```python
from build123d import *

# Parameters (mm, degrees)
F1_DEPTH  = 15.4
F3_DEPTH  = 5.4
F5_DEPTH  = 2
F6_R      = 6.7
F7_DEPTH  = 2
F9_DEPTH  = 8.7
F10_R     = 1.25
F11_DEPTH = 1
F12_R     = 2.85
F13_DEPTH = 3
F14_R     = 2.7
F15_DEPTH = 3
F16_R     = 1
F17_DEPTH = 5
F18_R     = 1.7
F18_R_2   = 1
F19_DEPTH = 3


with BuildPart() as f1:
    # F0 (on Top) → F1 (new body)
    with BuildSketch(Plane.XY):
        with BuildLine():
            Line((-22.9, -27.9), (22.9, -27.9))
            ThreePointArc((22.9, -27.9), (26.4355339059, -26.4355339059), (27.9, -22.9))
            Line((27.9, -22.9), (27.9, 22.9))
            ThreePointArc((27.9, 22.9), (26.4355339059, 26.4355339059), (22.9, 27.9))
            Line((22.9, 27.9), (-22.9, 27.9))
            ThreePointArc((-22.9, 27.9), (-26.4355339059, 26.4355339059), (-27.9, 22.9))
            Line((-27.9, 22.9), (-27.9, -22.9))
            ThreePointArc((-27.9, -22.9), (-26.4355339059, -26.4355339059), (-22.9, -27.9))
        make_face()
    extrude(amount=F1_DEPTH)

    # F2 (on face) → F3 (cut)
    with BuildSketch(Plane(origin=(0, 0, 0), x_dir=(1, 0, 0), z_dir=(0, 0, -1))):
        with BuildLine():
            Line((27.9, -11.9), (-27.9, -11.9))
            Line((-27.9, -11.9), (-27.9, -22.9))
            ThreePointArc((-27.9, -22.9), (-26.4355339059, -26.4355339059), (-22.9, -27.9))
            Line((-22.9, -27.9), (22.9, -27.9))
            ThreePointArc((22.9, -27.9), (26.4355339059, -26.4355339059), (27.9, -22.9))
            Line((27.9, -22.9), (27.9, -11.9))
        make_face()
    extrude(amount=-F3_DEPTH, mode=Mode.SUBTRACT)

    # F4 (on face) → F5 (cut)
    with BuildSketch(Plane(origin=(0, 0, 0), x_dir=(1, 0, 0), z_dir=(0, 0, -1))):
        with BuildLine():
            Line((27.9, -11.9), (27.9, 5.5))
            Line((27.9, 5.5), (19.5, 5.5))
            ThreePointArc((19.5, 5.5), (13.0653282912, 2.8346717088), (10.4, -3.6))
            Line((10.4, -3.6), (10.4, -11.9))
            Line((10.4, -11.9), (27.9, -11.9))
        make_face()
    extrude(amount=-F5_DEPTH, mode=Mode.SUBTRACT)

    # F6 (on face) → F7 (join)
    with BuildSketch(Plane(origin=(0, 0, 2), x_dir=(1, 0, 0), z_dir=(0, 0, -1))):
        with Locations((19.5, -3.6)):
            Circle(F6_R)
    extrude(amount=F7_DEPTH)

    # F8 (on face) → F9 (cut)
    with BuildSketch(Plane(origin=(0, 0, 5.4), x_dir=(1, 0, 0), z_dir=(0, 0, -1))):
        with BuildLine():
            Line((8, -26.6), (21.6, -26.6))
            ThreePointArc((21.6, -26.6), (25.1355339059, -25.1355339059), (26.6, -21.6))
            Line((26.6, -21.6), (26.6, -12.4))
            Line((26.6, -12.4), (-26.6, -12.4))
            Line((-26.6, -12.4), (-26.6, -21.6))
            ThreePointArc((-26.6, -21.6), (-25.1355339059, -25.1355339059), (-21.6, -26.6))
            Line((-21.6, -26.6), (-8, -26.6))
            Line((-8, -26.6), (-8, -26.55))
            ThreePointArc((-8, -26.55), (-7.8096194078, -26.0903805922), (-7.35, -25.9))
            Line((-7.35, -25.9), (7.35, -25.9))
            ThreePointArc((7.35, -25.9), (7.8096194078, -26.0903805922), (8, -26.55))
            Line((8, -26.55), (8, -26.6))
        make_face()
    extrude(amount=-F9_DEPTH, mode=Mode.SUBTRACT)

    # F10 (on face) → F11 (cut)
    with BuildSketch(Plane(origin=(0, 0, 0), x_dir=(1, 0, 0), z_dir=(0, 0, -1))):
        with Locations((19.5, -3.6)):
            Circle(F10_R)
    extrude(amount=-F11_DEPTH, mode=Mode.SUBTRACT)

    # F12 (on face) → F13 (join)
    with BuildSketch(Plane.XY.offset(15.4)):
        Circle(F12_R)
    extrude(amount=F13_DEPTH)

    # F14 (on face) → F15 (join)
    with BuildSketch(Plane.XY.offset(18.4)):
        Circle(F14_R)
    extrude(amount=F15_DEPTH)

    # F16 (on face) → F17 (cut)
    with BuildSketch(Plane.XY.offset(21.4)):
        Circle(F16_R)
    extrude(amount=-F17_DEPTH, mode=Mode.SUBTRACT)

    # F18 (on face) → F19 (join)
    with BuildSketch(Plane.XY.offset(21.4)):
        Circle(F18_R)
        Circle(F18_R_2, mode=Mode.SUBTRACT)
    extrude(amount=F19_DEPTH)


solid = f1.part
```
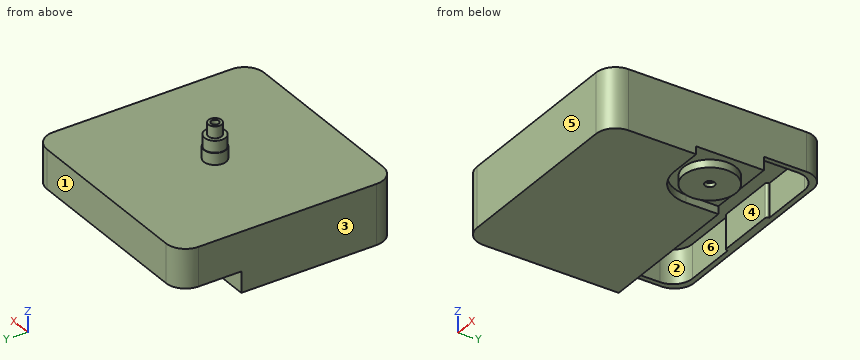
Check sheet for the modelled part. Datum: model origin and axes. Units: mm. Face numbers are marked on the shaded views. A direction names the side the tool comes from. Coordinates: 2 decimals unless noted, no trailing zeros. Order: outer loops, then holes, each group sorted by start corner. A loop starts at its lowest first (then second) coordinate and runs counter-clockwise, first axis right, second up. Notation, with made-up numbers: M -11,-28.5 L 27,-28.5 A12 cw 27,-8.5 Z; hole C -13.75,34 d7. An arc over 180 degrees is marked long. Write each question's results on one line, items separated by ' | '. Start each with the question number.
1. Access from +Z, -Z, +X, -X, +Y, -Y to the whole of each face (thin tool, end or side, straight path). Record for the marked faces 5 and 6.
2. Material ranges on probe 1 along Y at (x, z) = (19.5, 0.7); probe 2 along Y at (x, z) = (-9, 10); probe 3 along Y at (x, z) = (0, 20.75), recorded low to high.
3. Go/stop test with flat-tipped pins: P1, Ø7, axis at x = 9, y = 17.5, coming from the -Z side; P2, Ø0.7, axis at x = 19, y = 3.5, coming from the -Z side; P3, Ø12, axis at x = 3.5, y = -7, coming from the +Z side. Record where each tip stops, or that it passes through.
4. Cross-section at A-A on z = 9.25. Record the cut outline in (x, y).
5. Mould release check, pull along X, two halves, no side actions. Record for the marked faces 1, 2, 3 and 4: +X half, -X half, draft (parallel to the pull), parting line (faces both ways), or undercut.
6. Cross-section at C-C on y = -4. Record the cut outline in (x, z) (3 decimals), and give its area (3 significant figures).
7. Cross-section at D-D on x = 0. Record the cut outline in (y, z), and give its area (3 significant figures).
8. Cross-section at B-B on x = -16.5. Record the cut outline in (y, z).
Checks:
1) face 5: +Z, -Z, +X, -X, -Y | face 6: -Z
2) probe 1: y = -27.9 to -5.5, -3.1 to 2.35, 4.85 to 10.3 | probe 2: y = -27.9 to 12.4, 26.6 to 27.9 | probe 3: y = -2.7 to -1, 1 to 2.7
3) P1: stops at z = 14.1 | P2: stops at z = 1 | P3: stops at z = 21.4
4) outline: M -27.9,-22.9 A5 ccw -22.9,-27.9 L 22.9,-27.9 A5 ccw 27.9,-22.9 L 27.9,22.9 A5 ccw 22.9,27.9 L -22.9,27.9 A5 ccw -27.9,22.9 Z; hole M -26.6,12.4 L 26.6,12.4 L 26.6,21.6 A5 ccw 21.6,26.6 L 8,26.6 L 8,26.55 A0.65 cw 7.35,25.9 L -7.35,25.9 A0.65 cw -8,26.55 L -8,26.6 L -21.6,26.6 A5 ccw -26.6,21.6 Z
5) face 1: draft | face 2: undercut | face 3: -X half | face 4: undercut
6) outline: M -27.9,0 L 14.495,0 L 14.495,2 L 27.9,2 L 27.9,15.4 L -27.9,15.4 Z | area: 833 mm²
7) outline: M -27.9,0 L 11.9,0 L 11.9,5.4 L 12.4,5.4 L 12.4,14.1 L 25.9,14.1 L 25.9,5.4 L 27.9,5.4 L 27.9,15.4 L 2.85,15.4 L 2.85,18.4 L 2.7,18.4 L 2.7,21.4 L 1.7,21.4 L 1.7,24.4 L 1,24.4 L 1,16.4 L -1,16.4 L -1,24.4 L -1.7,24.4 L -1.7,21.4 L -2.7,21.4 L -2.7,18.4 L -2.85,18.4 L -2.85,15.4 L -27.9,15.4 Z | area: 683 mm²
8) outline: M -27.9,0 L 11.9,0 L 11.9,5.4 L 12.4,5.4 L 12.4,14.1 L 26.6,14.1 L 26.6,5.4 L 27.9,5.4 L 27.9,15.4 L -27.9,15.4 Z
